Part model, mm, in its own coordinate system. Face numbers are marked on the shaded views. A direction names the side the tool comes from. Round coordinates to 2 decimals unless told otherwise and drop trailing zeros. Loops run counter-clockwise (first coordinate to the right, second up) from the corner with the lowest first, then second, coordinate; pieces in that order, holes last.
(1) Cut at B-B on x = 92.5. List the corners of the cut face in (y, z) (3 decimals).
(2) Cut at A-A on y = 47. List the corners of the cut face in (x, z) (3 decimals), then the cut area to 3 significant figures.
(3) Probe probe 1 along X at (y, z) = (-1, -1.5) (3 decimals); probe 2 along Z at (x, y) = (73.5, -11) (3 decimals); probe 3 along Z at (x, y) = (-29, -50) (3 decimals). List the from-to ranges inside material, lowest first.
(4) Flat gauge pins, fed straight in: pin 1 (6 mm diameter, centred on y = 18.5, z = 27, fed in from +X); pin 2 (5 mm diameter, centred on y = -20.5, z = 14.5, fed in from -X) (3 decimals); pin 3 (6 mm diameter, centred on x = 83.5, z = 48.5, fed in from +Y). Where does each tip first touch, or does it go through?
(5) Tool access for the marked faces 1, 2, 3, 4 and 5: list every direction of +Z, -Z, +X, -X, +Y, -Y with a clear straight run to the whole face (end or side of a thin tool).
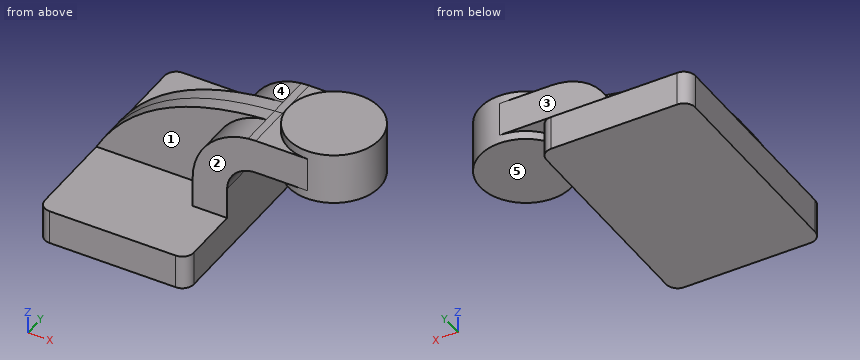
from build123d import *

# Parameters (mm, degrees)
F1_DEPTH = 63.5
F2_DEPTH = 25.4
F3_DEPTH = 7.9375
F0_W     = 25.4
F0_H     = 19.05
F4_DEPTH = 25.4
F6_R     = 6.35


with BuildPart() as f1:
    # F0 (on Front) → F1 (new body, symmetric)
    with BuildSketch(Plane.XZ):
        Polygon((22.225, 9.525), (-41.275, 9.525), (-41.275, -9.525), (41.275, -9.525), (41.275, 9.525), align=None)
    extrude(amount=F1_DEPTH, both=True)

    # F0 (on Front) → F2 (join, symmetric)
    with BuildSketch(Plane.XZ):
        with BuildLine():
            Line((22.225, 27.0002), (22.225, 9.525))
            Line((22.225, 9.525), (41.275, 9.525))
            Line((41.275, 9.525), (41.275, 27.0002))
            ThreePointArc((41.275, 27.0002), (45.92468, 38.22552), (57.15, 42.8752))
            Line((57.15, 42.8752), (60.325, 42.8752))
            Line((60.325, 42.8752), (60.325, 61.9252))
            Line((60.325, 61.9252), (57.15, 61.9252))
            add(Edge.make_bspline(
                [(52.876999, 61.662818), (54.307987, 61.76468), (55.732814, 61.851718), (57.15, 61.9252)],
                knots=[107.106385, 107.106385, 107.106385, 107.106385, 111.504536, 111.504536, 111.504536, 111.504536], degree=3))
            ThreePointArc((52.876999, 61.662818), (30.987143, 50.135898), (22.225, 27.0002))
        make_face()
    extrude(amount=F2_DEPTH, both=True)

    # F0 (on Front) → F3 (join, symmetric)
    with BuildSketch(Plane.XZ):
        with BuildLine():
            add(Edge.make_bspline(
                [(-41.275, 9.525), (-20.473646, 47.910034), (18.028728, 59.18221), (52.876999, 61.662818)],
                knots=[0, 0, 0, 0, 107.106385, 107.106385, 107.106385, 107.106385], degree=3))
            Line((-41.275, 9.525), (22.225, 9.525))
            Line((22.225, 9.525), (22.225, 27.0002))
            ThreePointArc((22.225, 27.0002), (30.987143, 50.135898), (52.876999, 61.662818))
        make_face()
    extrude(amount=F3_DEPTH, both=True)

    # F0 (on Front) → F4 (join, symmetric)
    with BuildSketch(Plane.XZ):
        with Locations((73.025, 52.4002)):
            Rectangle(F0_W, F0_H)
    extrude(amount=F4_DEPTH, both=True)

    # F0 (on Front) → F5 (revolve)
    with BuildSketch(Plane.XZ):
        Polygon((85.725, 66.675), (85.725, 61.9252), (85.725, 42.8752), (85.725, 38.1), (111.125, 38.1), (111.125, 66.675), align=None)
    revolve(axis=Axis((85.725, 0, 52.3875), (0, 0, -1)))

    # F6
    f6_edges = [f1.edges().sort_by_distance(p)[0] for p in [
        (41.275, -63.5, 0),
        (41.275, 63.5, 0),
        (-41.275, 63.5, 0),
        (-41.275, -63.5, 0),
    ]]
    fillet(f6_edges, radius=F6_R)


solid = f1.part
Final values:
1. outline: (-24.48, 38.1) - (24.48, 38.1) - (24.48, 66.675) - (-24.48, 66.675) - close
2. outline: (-41.275, -9.525) - (41.275, -9.525) - (41.275, 9.525) - (-41.275, 9.525) - close
2. area: 1,570 mm2
3. probe 1: x = -41.275 to 41.275
3. probe 2: z = 38.1 to 66.675
3. probe 3: z = -9.525 to 9.525
4. pin 1: stops at x = 41.56
4. pin 2: stops at x = 22.225
4. pin 3: stops at y = 25.4
5. face 1: +Z, -X, -Y
5. face 2: +Z, +X, -X, -Y
5. face 3: +Z, +X, -X, +Y
5. face 4: +Z, -X, +Y
5. face 5: -Z, +X, +Y, -Y
